For this review, take the finished solid that the model builds, in its own axes (mm). Round coordinates to 2 decimals unless told otherwise and drop trailing zeros. Loops run counter-clockwise (first coordinate to the right, second up) from the corner with the lowest first, then second, coordinate; pieces in that order, holes last. Notation, with made-up numbers: (3, 74) -> (27, 74) arc R25 cw to (27, 96) -> close; hole circle Ø9 at (-21.75, 17). An arc over 180 degrees is marked (long way). One line per question, with ' | ' between items. Start each with the question number.
1. For pin 1 Ø5 at (y, z) = (-2, 10.5) entering from -X; pin 2 Ø4 at (y, z) = (-3, 6) entering from +X, all flat-tipped, find the tip position at first contact; note any pin that passes through.
2. Consider section A-A (y = -16.5). Write out the cut boundary in (x, z), and give its area (3 significant figures).
3. Wall thickness on line 1 along Y through (x, z) = (76.2, 7.75); line 2 along X through (y, z) = (53, 4.5); line 3 along Y through (x, z) = (75, 7.5): over which ranges is each line inside the solid? List them lowest first.
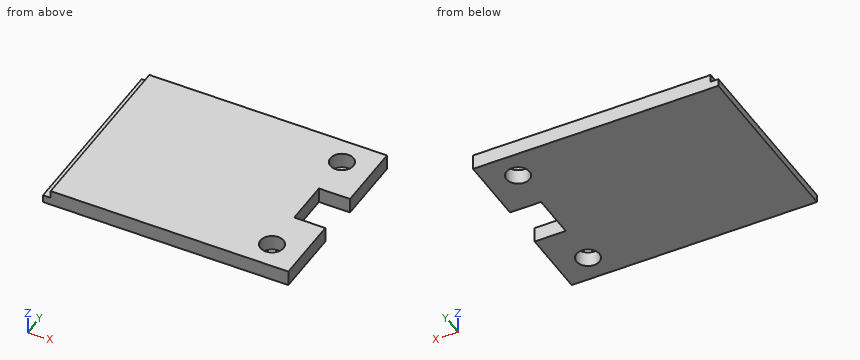
```python
from build123d import *

# Parameters (mm, degrees)
F0_R     = 9.525
F1_DEPTH = 12.7
F2_W     = 6.35
F2_H     = 6.35
F3_DEPTH = 152.401


with BuildPart() as f1:
    # F0 (on Top) → F1 (new body)
    with BuildSketch(Plane.XY):
        Polygon((101.6, 76.2), (-101.6, 76.2), (-101.6, -76.2), (101.6, -76.2), (101.6, -19.05), (75.863957, -19.05), (75.863957, 19.05), (101.6, 19.05), align=None)
        with Locations((76.2, -53.975)):
            Circle(F0_R, mode=Mode.SUBTRACT)
        with Locations((76.2, 53.975)):
            Circle(F0_R, mode=Mode.SUBTRACT)
    extrude(amount=F1_DEPTH)

    # F2 (on face) → F3 (cut, through all)
    with BuildSketch(Plane.XZ.offset(76.2)):
        with Locations((-98.425, 9.525)):
            Rectangle(F2_W, F2_H)
    extrude(amount=-F3_DEPTH, mode=Mode.SUBTRACT)


solid = f1.part
```
Answer block:
1) pin 1: stops at x = -95.25 | pin 2: stops at x = 75.86
2) outline: (-101.6, 0) -> (75.86, 0) -> (75.86, 12.7) -> (-95.25, 12.7) -> (-95.25, 6.35) -> (-101.6, 6.35) -> close | area: 2,210 mm2
3) line 1: y = -76.2 to -63.5, -44.45 to -19.05, 19.05 to 44.45, 63.5 to 76.2 | line 2: x = -101.6 to 66.73, 85.67 to 101.6 | line 3: y = -76.2 to -63.42, -44.53 to 44.53, 63.42 to 76.2
